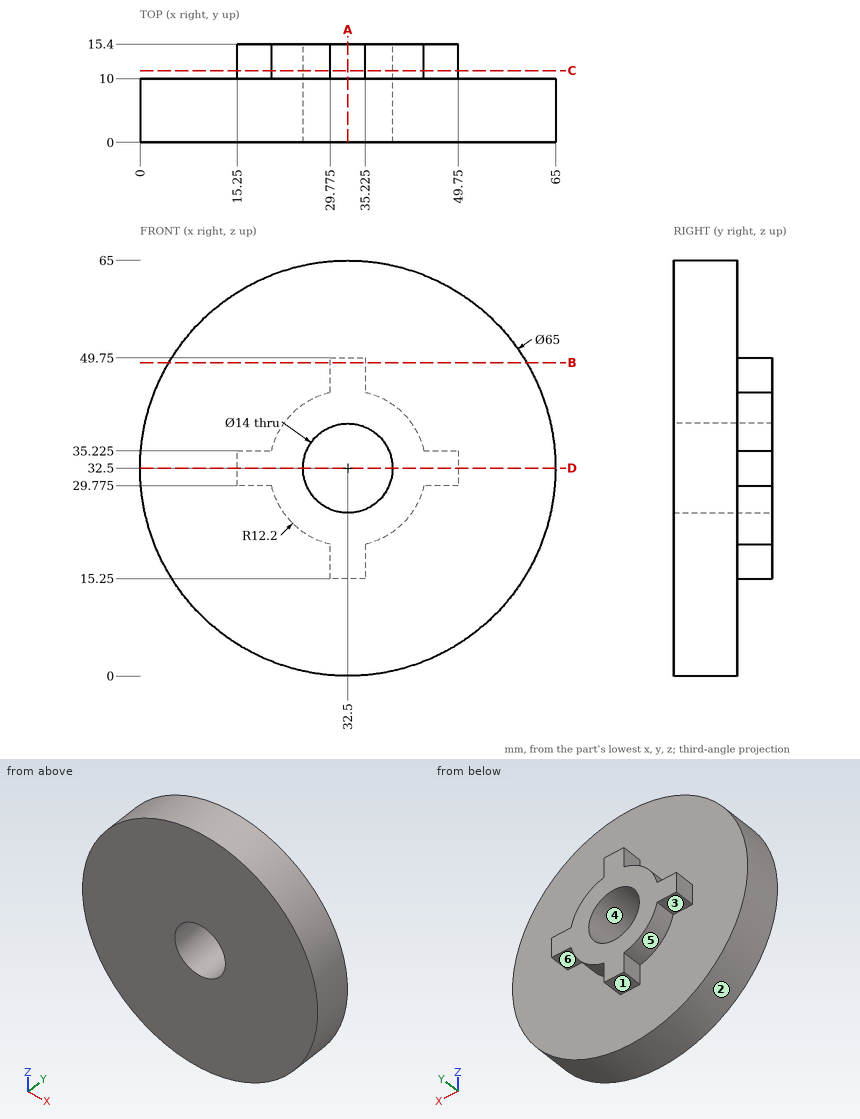
Check sheet for the drawn part. Datum: minimum x, y, z corner. Units: mm. A direction names the side the tool comes from. Round coordinates to 2 decimals unless told otherwise and drop trailing zeros. Loops run counter-clockwise (first coordinate to the right, second up) from the corner with the lowest first, then second, coordinate; pieces in that order, holes last. Notation, with made-up numbers: (54, -6.75) - (74, -6.75) arc R9 ccw to (74, 8.25) - close; hole circle Ø7 at (54, 54). An arc over 180 degrees is marked (long way). Answer as a JSON object with one key per item and string values. Group by question number.
Q1. Sectioned sample at C-C, the plane y = 11.25. Enter the section's corners in (x, z) (3 decimals).
Q2. Set-up check for the marked faces 1, 2 and 3: record each of +Z, -Z, +X, -X, +Y, -Y from which the full face is reachable in a straight line by a thin tool's end or side.
Q3. Sectioned sample at A-A, the plane x = 32.5. Enter the section's corners in (y, z).
Q4. Scan lines: line 1 along X through (y, z) = (11, 32.5); line 2 along X through (y, z) = (4.5, 32.5); line 3 along Y through (x, z) = (18.5, 11). Record each from-to range of solid material in increasing order. Write a range as [from, to].
Q5. Mould release check, pull along X, two halves, no side actions. Record for the marked faces 4, 5 and 6: released by +X, released by -X, zero draft, split by the parting line, or undercut.
Q6. Gauge pin test, flat ends, axial feed: P1, Ø5, axis at x = 39, y = 13, coming from the -Z side; P2, Ø4.5, axis at y = 13.5, z = 48, coming from the -X side (3 decimals); P3, Ø8, axis at x = 24.5, y = 7, coming from the -Z side. Record the tip position at first contact, or that the pin passes through.
Q7. Sectioned sample at B-B, the plane z = 49. Enter the section's corners in (x, y) (3 decimals).
Q8. Sectioned sample at D-D, the plane z = 32.5. Enter the section's corners in (x, y), plus the area to 3 significant figures.
Solution:
{
 "1": {"outline": "(15.25, 29.775) - (20.608, 29.775) arc R12.2 ccw to (29.775, 20.608) - (29.775, 15.25) - (35.225, 15.25) - (35.225, 20.608) arc R12.2 ccw to (44.392, 29.775) - (49.75, 29.775) - (49.75, 35.225) - (44.392, 35.225) arc R12.2 ccw to (35.225, 44.392) - (35.225, 49.75) - (29.775, 49.75) - (29.775, 44.392) arc R12.2 ccw to (20.608, 35.225) - (15.25, 35.225) - close; hole circle Ø14 at (32.5, 32.5)"},
 "2": {"face 1": "-Z, +X, -X, +Y", "face 2": "+Y, -Y", "face 3": "-Z, -X, +Y"},
 "3": {"outline": "(0, 0) - (10, 0) - (10, 15.25) - (15.4, 15.25) - (15.4, 25.5) - (0, 25.5) - close; (0, 39.5) - (15.4, 39.5) - (15.4, 49.75) - (10, 49.75) - (10, 65) - (0, 65) - close"},
 "4": {"line 1": "x = [15.25, 25.5], [39.5, 49.75]", "line 2": "x = [0, 25.5], [39.5, 65]", "line 3": "y = [0, 10]"},
 "5": {"face 4": "undercut", "face 5": "released by -X", "face 6": "zero draft"},
 "6": {"P1": "stops at z = 20.97", "P2": "stops at x = 29.775", "P3": "stops at z = 0.25"},
 "7": {"outline": "(4.5, 0) - (60.5, 0) - (60.5, 10) - (35.225, 10) - (35.225, 15.4) - (29.775, 15.4) - (29.775, 10) - (4.5, 10) - close"},
 "8": {"outline": "(0, 0) - (25.5, 0) - (25.5, 15.4) - (15.25, 15.4) - (15.25, 10) - (0, 10) - close; (39.5, 0) - (65, 0) - (65, 10) - (49.75, 10) - (49.75, 15.4) - (39.5, 15.4) - close", "area": "621 mm²"}
}
